Autodesk Inventor part; units mm, degrees
ref_plane "YZ Plane" through (0, 0, 0) normal (1, 0, 0) x (0, 1, 0)
ref_plane "XZ Plane" through (0, 0, 0) normal (0, 1, 0) x (-1, 0, 0)
ref_plane "XY Plane" through (0, 0, 0) normal (0, 0, 1) x (1, 0, 0)
sketch "Sketch1" plane through (0, 0, 0) normal (0, 1, 0) x (-1, 0, 0)
  line L0 (0, 0) -> (-40, 0)
  line L1 (-40, 0) -> (-40, -30)
  line L2 (-40, -30) -> (0, -30)
  line L3 (0, -30) -> (0, 0)
  dimension "d0" = 30
  dimension "d1" = 40
extrude "Extrusion1" add sketch "Sketch1" along normal blind 3
sketch "Sketch2" plane through (0, 3, 0) normal (0, 1, 0) x (1, 0, 0)
  circle A0 centre (20, 15) radius 7.5
  line L0 (0, 30) -> (0, 0)
  line L1 (0, 0) -> (40, 0)
  dimension "d4" = 15
  dimension "d5" = 20
  dimension "d6" = 15
extrude "Extrusion2" cut sketch "Sketch2" against normal blind 3
sketch "Sketch3" plane through (0, 3, 0) normal (0, 1, 0) x (1, 0, 0)
  circle A0 centre (20, 15) radius 7.5
  circle A1 centre (20, 15) radius 7.5
  circle A2 centre (20, 15) radius 12.8
  point P0 (0, 0)
  dimension "d9" = 25.6
extrude "Extrusion3" add sketch "Sketch3" along normal blind 2
sketch "Sketch4" plane through (0, 0, 0) normal (0, -1, 0) x (1, 0, 0)
  circle A0 centre (5, -25) radius 2.368
  circle A1 centre (5, -5) radius 2.5
  circle A2 centre (35, -25) radius 2.5
  circle A3 centre (35, -5) radius 2.5
  circle A4 centre (20, -15) radius 7.5
  point P0 (0, 0)
  dimension "d12" = 5
  dimension "d13" = 5
  dimension "d14" = 5
  dimension "d15" = 15
  dimension "d16" = 10
  dimension "d17" = 10
  dimension "d18" = 15
  dimension "d19" = 15
  dimension "d20" = 15
  dimension "d21" = 10
  dimension "d22" = 10
extrude "Extrusion4" cut sketch "Sketch4" against normal blind 2 contours A0 | A1 | A2 | A3
chamfer "Chamfer1" distance 4 angle 45 4 edges at (40, 1.5, 0) (40, 1.5, -30) (0, 1.5, 0) (0, 1.5, -30)
sketch "Sketch5" plane through (0, 3, 0) normal (0, 1, 0) x (1, 0, 0)
  line L0 (36, 30) -> (4, 30)
  line L1 (17, 30) -> (23, 30)
  line L2 (23, 30) -> (23, 32)
  line L3 (23, 32) -> (17, 32)
  line L4 (17, 32) -> (17, 30)
  line L5 (17, 0) -> (23, 0)
  line L6 (23, 0) -> (23, -2)
  line L7 (23, -2) -> (17, -2)
  line L8 (17, -2) -> (17, 0)
  line L9 (0, 26) -> (0, 4)
  line L10 (4, 0) -> (36, 0)
  point P0 (0, 0)
  dimension "d28" = 6
  dimension "d29" = 17
  dimension "d30" = 2
  dimension "d31" = 6
  dimension "d32" = 17
  dimension "d33" = 2
  dimension "d34" = 0
  dimension "d35" = 2
extrude "Extrusion5" add sketch "Sketch5" against normal blind 3
sketch "Sketch6" plane through (20, 5, -15) normal (0, 1, 0) x (1, 0, 0)
  circle A0 centre (0, 0) radius 9.55
  circle A1 centre (0, 0) radius 7.9
  point P0 (-20, -15)
  dimension "d38" = 15.8
  dimension "d39" = 19.1
extrude "Extrusion6" cut sketch "Sketch6" against normal blind 0.7
fillet "Fillet1" radius 0.8 2 edges at (12.1, 4.3, -15) (10.45, 4.3, -15)
properties part number "chamber_top"
Work out the finished part from the listing and answer in its coordinate system (mm). A direction names the side the tool comes from. Give positions to 0.01 mm unless a question says otherwise; leave off trailing zeros. Loops run counter-clockwise (first coordinate to the right, second up) from the corner with the lowest first, then second, coordinate; pieces in that order, holes last. Notation, with made-up numbers: M 35,-27 L 54,-27 A24 cw 54,12 Z; hole C 85.5,36 d7. An arc over 180 degrees is marked long. Use CSV: the item, a comma, the result in double quotes.
1) Given P1, Ø2.5, axis at x = 6, z = -5, coming from the -Y side; P2, Ø6, axis at x = 35, z = -5, coming from the +Y side; P3, Ø1.6, axis at y = 2, z = 0.5, coming from the +X side; P4, Ø2, axis at y = 1, z = -5.5, coming from the -X side, each flat-ended and moving along its own axis, determine where each tip first touches the part or whether it passes through.
Answer:
P1,"y = 2"
P2,"y = 3"
P3,"x = 36.3"
P4,"x = 0"
2) Find section C-C on z = -5. Write down the section's boundary in (x, y), plus the area to 3 significant figures.
Answer:
outline,"M 0,0 L 2.5,0 L 2.5,2 L 7.5,2 L 7.5,0 L 32.5,0 L 32.5,2 L 37.5,2 L 37.5,0 L 40,0 L 40,3 L 27.99,3 L 27.99,5 L 12.01,5 L 12.01,3 L 0,3 Z"
area,"132 mm^2"
3) Consider L1, parallel to Z at x = 35, y = 1.35; L2, parallel to Z at x = 5, y = 0.75; L3, parallel to X at y = 1.1, z = -15. Determine where each line is inside the solid, lowest interval first.
Answer:
L1,"-30 to -27.5, -22.5 to -7.5, -2.5 to 0"
L2,"-30 to -27.37, -22.63 to -7.5, -2.5 to 0"
L3,"0 to 12.5, 27.5 to 40"
4) Find section A-A on z = -15. Write down the section's boundary in (x, y), plus the area to 3 significant figures.
Answer:
outline,"M 0,0 L 12.5,0 L 12.5,5 L 12.09,5 A0.8 cw 11.3,4.3 L 11.25,4.3 A0.8 cw 10.46,5 L 7.2,5 L 7.2,3 L 0,3 Z; M 27.5,0 L 40,0 L 40,3 L 32.8,3 L 32.8,5 L 29.54,5 A0.8 cw 28.75,4.3 L 28.7,4.3 A0.8 cw 27.91,5 L 27.5,5 Z"
area,"94.4 mm^2"
5) Determine the mould class of faces 6 (the cylindrical face through (9.842, 3.986, -22.789)), 7 (the cylindrical face through (37.31, 0.99, -5.96)), 8 (the flat face through (11, 1, -30)) for opening direction Z: released by +Z, released by -Z, zero draft, split by the parting line, or undercut.
Answer:
face 6,"split by the parting line"
face 7,"undercut"
face 8,"released by -Z"
6) Find section B-B on x = 35. Write down the section's boundary in (y, z).
Answer:
outline,"M 0,-30 L 3,-30 L 3,0 L 0,0 L 0,-2.5 L 2,-2.5 L 2,-7.5 L 0,-7.5 L 0,-22.5 L 2,-22.5 L 2,-27.5 L 0,-27.5 Z"
7) Which of the six approach directions +Z, -Z, +X, -X, +Y, -Y give full straight-line access (tool end or side, diameter ignored) to faces 1 (the cylindrical face through (7.385, 0.986, -4.249)), 2 (the flat face through (10, 1, 0)), 3 (the flat face through (0, 1, -15)), 4 (the flat face through (23, 2, 1)), 5 (the flat face through (30, 1, -30))?
Answer:
face 1,"-Y"
face 2,"+Z, -X, +Y, -Y"
face 3,"+Z, -Z, -X, +Y, -Y"
face 4,"+Z, +X, +Y, -Y"
face 5,"-Z, +X, +Y, -Y"
8) Find section D-D on x = 5. Write down the section's boundary in (y, z), plus the area to 3 significant figures.
Answer:
outline,"M 0,-30 L 3,-30 L 3,0 L 0,0 L 0,-2.5 L 2,-2.5 L 2,-7.5 L 0,-7.5 L 0,-22.63 L 2,-22.63 L 2,-27.37 L 0,-27.37 Z"
area,"70.5 mm^2"
